Design review of the part shown in the three views and the two pictorial views. Dimensions are in mm from the part's minimum x, y and z. A direction names the side the tool comes from. Coordinates: 2 decimals unless noted, no trailing zeros. Loops run counter-clockwise (first coordinate to the right, second up) from the corner with the lowest first, then second, coordinate; pieces in that order, holes last. Notation, with made-up numbers: (-25.75, 23) - (-18.75, 23) arc R35 ccw to (-18.75, 58) - close; hole circle Ø10 at (-3.75, 65). An arc over 180 degrees is marked (long way). One line per question, with ' | ' between items.
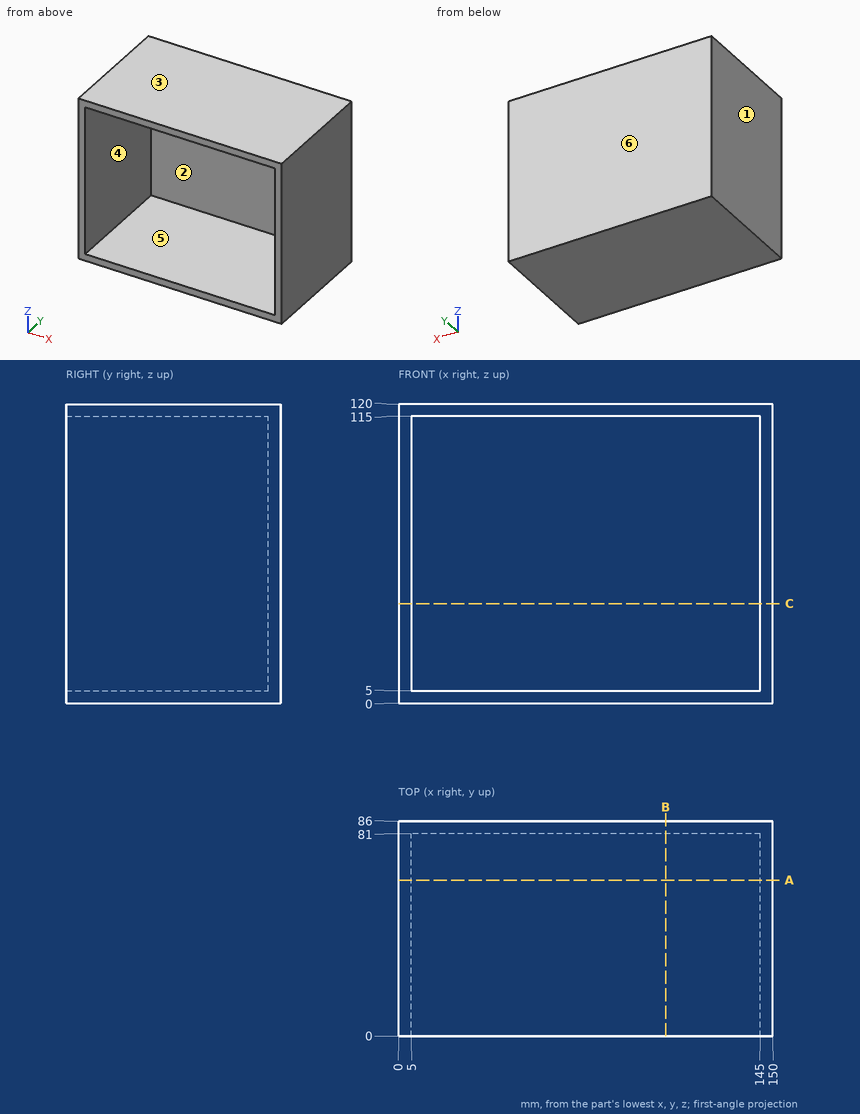
Q1. Take a section at C-C (z = 40). Give the boundary of the cut face in (x, y).
Returned:
outline: (0, 0) - (5, 0) - (5, 81) - (145, 81) - (145, 0) - (150, 0) - (150, 86) - (0, 86) - close
Q2. Tool access review of the marked faces 5 and 6: name each direction out of +Z, -Z, +X, -X, +Y, -Y from which nothing blocks a thin tool from reaching the whole face with its end or side.
Returned:
face 5: -Y | face 6: +Z, -Z, +X, -X, +Y
Q3. Draft analysis for pull direction Z (two halves, no side actions). For the marked faces 1, 2, 3 and 4, state which applies: +Z half, -Z half, draft (parallel to the pull), parting line (faces both ways), or undercut.
Returned:
face 1: draft | face 2: undercut | face 3: +Z half | face 4: undercut
Q4. To check wall thickness, follow line 1 along Z through (x, y) = (135.5, 18); line 2 along X through (y, z) = (38.5, 102); line 3 along Y through (x, z) = (81.5, 86). State the ranges of each line that lie inside material, in increasing order.
Returned:
line 1: z = 0 to 5, 115 to 120 | line 2: x = 0 to 5, 145 to 150 | line 3: y = 81 to 86
Q5. For pin 1 (4 mm diameter, centred on x = 96.5, z = 99.5, fed in from -Y), flat-tipped, find the tip position at first contact; note if it passes through.
Returned:
pin 1: stops at y = 81
Q6. Take a section at A-A (y = 62.5). Give the boundary of the cut face in (x, z).
Returned:
outline: (0, 0) - (150, 0) - (150, 120) - (0, 120) - close; hole (5, 5) - (145, 5) - (145, 115) - (5, 115) - close
Q7. Take a section at B-B (x = 107). Give the boundary of the cut face in (y, z), plus the area to 3 significant figures.
Returned:
outline: (0, 0) - (86, 0) - (86, 120) - (0, 120) - (0, 115) - (81, 115) - (81, 5) - (0, 5) - close | area: 1,410 mm²
